Build history of the part. All positions in model axes, mm. A direction names the side the tool comes from. Give positions to 0.01 mm unless a question says otherwise; leave off trailing zeros. Write each loop counter-clockwise with the first axis right and the second up, starting at its lowest first coordinate (ties: lowest second). Pieces come first, ordered by that corner, then holes. Notation, with made-up numbers: (-14.75, -14.5) -> (12.25, -14.5) arc R12 ccw to (12.25, 0.5) -> close; hole circle Ø1 at (-40, 69). An arc over 180 degrees is marked (long way). Put each result on its own line as item: value. Start each with the question number.
Item 1: Slice it at C-C, the plane y = -38.5. List the corners of the cut face in (x, z), plus the area to 3 significant figures.
Item 2: Drill centre lines: line 1 along Y through (x, z) = (-4, 43); line 2 along X through (y, z) = (-35.5, 51); line 3 along Y through (x, z) = (-4, 34.5). Where is each one in solid material? Low to high.
Item 3: Slice it at A-A, the plane x = 0.5. List the corners of the cut face in (y, z) (1 decimal).
Item 4: Flat gauge pins, fed straight in: pin 1 Ø2.5 at (x, z) = (-4, 26.5) entering from -Y; pin 2 Ø3 at (x, z) = (-0.5, 14.5) entering from +Y; pin 3 Ø4.5 at (x, z) = (-1, 36.5) entering from +Y. Where does each tip first touch, or does it go through?
Item 5: Slice it at D-D, the plane x = -6.5. List the corners of the cut face in (y, z), plus the area to 3 significant figures.
Item 6: Two-plate mould, pull along X, no slides. Class faces 1 (the flat face through (10, -22, 40)), 2 (the flat face through (4.19, -29.43, 56.85)), 3 (the flat face through (-7, 0, 51)), 4 (the flat face through (0, -6.1, 48)): pulls with the +X half, pulls with the -X half, needs draft (parallel to the pull), parting line crosses it, or undercut.
Item 7: Slice it at B-B, the plane z = 69.5. List the corners of the cut face in (x, y).
Item 8: Tool access for faces 5 (the flat face through (-4, -1.8, 51)), 6 (the flat face through (-5.5, -31, 58)), 7 (the flat face through (3.87, -33.38, 58.08)): list every direction of +Z, -Z, +X, -X, +Y, -Y with a clear straight run to the whole face (end or side of a thin tool).
```python
from build123d import *

# Parameters (mm, degrees)
PROFILE_START                   = -10
PROFILE_EXTRUDE_DEPTH           = 20
TOP_T_NUT_SLOT_CUT_DEPTH        = 122.194199002
FRONT_EDGE_CHAMFER_SIZE         = 10
FRONT_EDGE_CHAMFER_SIZE2        = 20
FRONT_T_NUT_SLOT_CUT_DEPTH      = 127.560696268
FRONT_T_NUT_SLOT_CUT_DEPTH_BACK = 95.470054


with BuildPart() as part:
    # Profile Sketch → Profile Extrude (new body)
    with BuildSketch(Plane(origin=(0, -25.324194998, 100.875319125), x_dir=(0, 1, 0), z_dir=(1, 0, 0)).offset(PROFILE_START)):
        Polygon((-42.410831921, -100.875319125), (15.324194998, -0.875319125), (25.324194998, -0.875319125), (25.324194998, -100.875319125), align=None)
    extrude(amount=PROFILE_EXTRUDE_DEPTH)

    # Top T-Nut Slot Sketch → Top T-Nut Slot Cut (cut, through all)
    with BuildSketch(Plane.XY.offset(100)):
        Polygon((-4.58, 0), (-3.13, -1.45), (-3.13, -1.8), (-5.5, -1.8), (-5.5, -3.44), (-2.84, -6.1), (2.84, -6.1), (5.5, -3.44), (5.5, -1.8), (3.13, -1.8), (3.13, -1.45), (4.58, 0), align=None)
    extrude(amount=-TOP_T_NUT_SLOT_CUT_DEPTH, mode=Mode.SUBTRACT)

    # Front Edge Chamfer
    front_edge_chamfer_edges = [part.edges().sort_by_distance(p)[0] for p in [
        (0, -67.735026919, 0),
    ]]
    front_edge_chamfer_side = [part.faces().sort_by_distance(p)[0] for p in [
        (0, -35.138756164, 0),
    ]]
    chamfer(front_edge_chamfer_edges, length=FRONT_EDGE_CHAMFER_SIZE, length2=FRONT_EDGE_CHAMFER_SIZE2, reference=front_edge_chamfer_side[0])

    # Front T-Nut Slot Sketch → Front T-Nut Slot Cut (cut, two sides: drawn at the far end of the back side and taken through both)
    with BuildSketch(Plane(origin=(20, 44.249147411, 68.679240139), x_dir=(-1, 0, 0), z_dir=(0, 0.5000000000000038, 0.8660254037844364)).offset(-FRONT_T_NUT_SLOT_CUT_DEPTH_BACK)):
        Polygon((15.42, 62.641519722), (16.87, 61.191519722), (16.87, 60.841519722), (14.5, 60.841519722), (14.5, 59.201519722), (17.16, 56.541519722), (22.84, 56.541519722), (25.5, 59.201519722), (25.5, 60.841519722), (23.13, 60.841519722), (23.13, 61.191519722), (24.58, 62.641519722), align=None)
    extrude(amount=FRONT_T_NUT_SLOT_CUT_DEPTH + FRONT_T_NUT_SLOT_CUT_DEPTH_BACK, mode=Mode.SUBTRACT)


solid = part.part
```
Values follow:
1. outline: (-10, 0) -> (10, 0) -> (10, 50.64) -> (4.58, 50.64) -> (3.13, 47.74) -> (3.13, 47.04) -> (5.5, 47.04) -> (5.5, 43.76) -> (2.84, 38.44) -> (-2.84, 38.44) -> (-5.5, 43.76) -> (-5.5, 47.04) -> (-3.13, 47.04) -> (-3.13, 47.74) -> (-4.58, 50.64) -> (-10, 50.64) -> close
1. area: 906 mm2
2. line 1: -42.24 to -40.83, -37.2 to -4.94, -1.8 to -0.58
2. line 2: -10 to -5.5, 5.5 to 10
2. line 3: -47.15 to -45.74, -42.11 to -4.94, -1.8 to -0.58
3. outline: (-57.7, 0) -> (-6.1, 0) -> (-6.1, 94.6) -> (-52.5, 14.3) -> (-57.7, 17.3) -> close
4. pin 1: y = -53.07
4. pin 2: y = -6.1
4. pin 3: y = -1.33
5. outline: (-57.74, 0) -> (0, 0) -> (0, 100) -> (-10, 100) -> (-57.74, 17.32) -> close
5. area: 3,800 mm2
6. face 1: pulls with the +X half
6. face 2: undercut
6. face 3: needs draft
6. face 4: undercut
7. outline: (-10, -27.61) -> (-4.58, -27.61) -> (-3.13, -25.93) -> (-3.13, -25.53) -> (-5.5, -25.53) -> (-5.5, -23.64) -> (-2.84, -20.57) -> (2.84, -20.57) -> (5.5, -23.64) -> (5.5, -25.53) -> (3.13, -25.53) -> (3.13, -25.93) -> (4.58, -27.61) -> (10, -27.61) -> (10, 0) -> (4.58, 0) -> (3.13, -1.45) -> (3.13, -1.8) -> (5.5, -1.8) -> (5.5, -3.44) -> (2.84, -6.1) -> (-2.84, -6.1) -> (-5.5, -3.44) -> (-5.5, -1.8) -> (-3.13, -1.8) -> (-3.13, -1.45) -> (-4.58, 0) -> (-10, 0) -> close
8. face 5: +Z, -Z
8. face 6: none
8. face 7: +Z, -Y
